Source: CAD feature listing. Evaluate the final solid. Frame: model axes, mm. A direction names the side the tool comes from. Give positions to 0.01 mm unless a question says otherwise; leave off trailing zeros. Write each loop counter-clockwise with the first axis right and the second up, starting at its lowest first coordinate (ties: lowest second). Pieces come first, ordered by that corner, then holes. Notation, with made-up numbers: (14, 53.25) -> (70, 53.25) arc R18 cw to (70, 60.25) -> close; hole circle Ø4 at (38, 78.5). An arc over 180 degrees is marked (long way). Write item = value, one per line.
Autodesk Inventor part; units mm, degrees
ref_plane "Work Plane1" through (18, 0, 0) normal (1, 0, 0) x (0, 1, 0)
ref_plane "Work Plane2" through (0, 0, 5) normal (0, 0, 1) x (1, 0, 0)
ref_plane "XZ Plane" through (0, 0, 0) normal (0, 1, 0) x (-1, 0, 0)
sketch "Sketch1" plane through (0, 0, 0) normal (0, 0, 1) x (1, 0, 0)
  circle A0 centre (0, 0) radius 20
  dimension "d0" = 40
extrude "Extrusion1" add sketch "Sketch1" along normal blind 25
shell "Shell1" thickness 5 removed faces 1 at (-2.364, 6.2334, 25)
fillet "Fillet1" radius 5 1 edges at (-15, 0, 5)
sketch "Sketch2" plane through (0, 0, 0) normal (1, 0, 0) x (0, 1, 0)
  line L0 (-28, 0) -> (28, 0)
  line L1 (0, -5) -> (0, 30)
  circle A0 centre (0, 20) radius 4
  line L2 (20, 25) -> (-20, 25)
  point P0 (0, 0)
  dimension "d5" = 8
  dimension "d6" = 5
extrude "Extrusion2" add sketch "Sketch2" along normal through all both and the other way through all
ref_plane "Work Plane1" through (18, 0, 0) normal (1, 0, 0) x (0, 1, 0)
sketch "Sketch3" plane through (18, 0, 0) normal (1, 0, 0) x (0, 1, 0)
  spline S0 degree 5 poles (4, 20) (4, 20.475) (3.9296, 20.9492) (3.7887, 21.4163) (3.5746, 21.8668) (3.0962, 22.5531) (2.8791, 22.8072) (2.6286, 23.0458) (2.3433, 23.263) (1.6847, 23.649) (1.3023, 23.8174) (0.8849, 23.938) (0.4453, 24) (-0.4453, 24) (-0.8849, 23.938) (-1.3023, 23.8174) (-1.6847, 23.649) (-2.3433, 23.263) (-2.6286, 23.0458) (-2.8791, 22.8072) (-3.0962, 22.5531) (-3.5746, 21.8668) (-3.7887, 21.4163) (-3.9296, 20.9492) (-4, 20.475) (-4, 19.6437) (-3.9603, 19.2875) (-3.881, 18.9346) (-3.7611, 18.5887) (-3.4806, 18.0102) (-3.3396, 17.7723) (-3.1752, 17.5422) (-2.9865, 17.3225) (-2.4836, 16.839) (-2.1457, 16.5837) (-1.7587, 16.3645) (-1.3265, 16.1959) (-0.4314, 15.9995) (0.0204, 15.9613) (0.4754, 15.9901) (0.9122, 16.0827) (1.662, 16.3427) (1.9854, 16.5006) (2.2787, 16.6866) (2.5408, 16.8939) (3.2793, 17.604) (3.6446, 18.1696) (3.8809, 18.7676) (4, 19.3828) (4, 20) knots 0 0 0 0 0 0 0.108769 0.108769 0.108769 0.108769 0.177598 0.177598 0.177598 0.177598 0.250135 0.250135 0.250135 0.250135 0.322672 0.322672 0.322672 0.322672 0.3915 0.3915 0.3915 0.3915 0.50027 0.50027 0.50027 0.50027 0.581861 0.581861 0.581861 0.581861 0.641459 0.641459 0.641459 0.641459 0.721814 0.721814 0.721814 0.721814 0.794745 0.794745 0.794745 0.794745 0.859101 0.859101 0.859101 0.859101 1 1 1 1 1 1
  point P0 (0, 0)
  dimension "d10" = 0
extrude "Extrusion3" cut sketch "Sketch3" along normal through all
mirror "Mirror1" about plane through (0, 0, 0) normal (1, 0, 0) of "Extrusion3"
ref_plane "Work Plane2" through (0, 0, 5) normal (0, 0, 1) x (1, 0, 0)
sketch "Sketch4" plane through (0, 0, 5) normal (0, 0, 1) x (1, 0, 0)
  circle A0 centre (0, 0) radius 15
  circle A1 centre (0, 0) radius 20
  circle A2 centre (0, 0) radius 19
  dimension "d14" = 1
extrude "Extrusion4" cut sketch "Sketch4" along normal blind 1 contours A1
pattern_linear "Rectangular Pattern1" count 3 spacing 2 along (0, 0, 1) of "Extrusion4"
properties part number "Piston" material "Steel, Carbon"
1) Cut plane A-A (z = 13.25). Return the cut outline in (x, y), then the cut area to 3 significant figures.
Computed:
outline = circle Ø40 at (0, 0); hole circle Ø30 at (0, 0)
area = 550 mm²
2) Cut plane D-D (y = 16.5). Return the cut outline in (x, z).
Computed:
outline = (-11.3, 0) -> (11.3, 0) -> (11.3, 5) -> (9.42, 5) -> (9.42, 6) -> (11.3, 6) -> (11.3, 7) -> (9.42, 7) -> (9.42, 8) -> (11.3, 8) -> (11.3, 9) -> (9.42, 9) -> (9.42, 10) -> (11.3, 10) -> (11.3, 25) -> (-11.3, 25) -> (-11.3, 10) -> (-9.42, 10) -> (-9.42, 9) -> (-11.3, 9) -> (-11.3, 8) -> (-9.42, 8) -> (-9.42, 7) -> (-11.3, 7) -> (-11.3, 6) -> (-9.42, 6) -> (-9.42, 5) -> (-11.3, 5) -> close
3) Cut plane C-C (z = 23). State how many separate pieces and enclosed holes the cut face has, then the cut area to 3 significant figures.
Computed:
separate_pieces = 1
enclosed_holes = 2
area = 687 mm²
4) Draft query along X for faces 3 (the cylindrical face through (-4.336, 19.524, 2.465)), 4 (the cylindrical face through (0.21, -0.521, 23.966)), 5 (the flat face through (3, 15, 25)). Return one class per face: pulls with the +X half, pulls with the -X half, needs draft (parallel to the pull), parting line crosses it, or undercut.
Computed:
face_3 = parting line crosses it
face_4 = undercut
face_5 = needs draft
5) Cut plane B-B (y = -17). Return the cut outline in (x, z), then the cut area to 3 significant figures.
Computed:
outline = (-10.54, 0) -> (10.54, 0) -> (10.54, 5) -> (8.49, 5) -> (8.49, 6) -> (10.54, 6) -> (10.54, 7) -> (8.49, 7) -> (8.49, 8) -> (10.54, 8) -> (10.54, 9) -> (8.49, 9) -> (8.49, 10) -> (10.54, 10) -> (10.54, 25) -> (-10.54, 25) -> (-10.54, 10) -> (-8.49, 10) -> (-8.49, 9) -> (-10.54, 9) -> (-10.54, 8) -> (-8.49, 8) -> (-8.49, 7) -> (-10.54, 7) -> (-10.54, 6) -> (-8.49, 6) -> (-8.49, 5) -> (-10.54, 5) -> close
area = 514 mm²
6) Access query for faces 1 (the cylindrical face through (-4.336, 19.524, 6.493)), 2 (the flat face through (18, -7, 7)). Directions: +Z, -Z, +X, -X, +Y, -Y. A direction counts if a zero-diameter tool reaches every point of the face in a straight line with its end or side. Return the directions, or none.
Computed:
face_1 = +Z, -Z
face_2 = none
7) Contact query for flat-ended pins moving along their axis: pin 1 (6 mm diameter, centred on y = -13.5, z = 14.5, fed in from -X); pin 2 (5 mm diameter, centred on y = 7.5, z = 10, fed in from -X); pin 3 (1 mm diameter, centred on x = -3.5, z = 12.5, fed in from +Y). Output: stop coordinate, or through.
Computed:
pin_1 = -17.02
pin_2 = -19.36
pin_3 = 19.77
8) Material intervals for L1, parallel to Z at x = -7.5, y = -18; L2, parallel to Y at x = 0, z = 15.75; L3, parallel to Y at x = -12.5, z = 16.75, sorted ascending.
Computed:
L1 = 0 to 5, 6 to 7, 8 to 9, 10 to 25
L2 = -20 to -15, 15 to 20
L3 = -15.61 to -8.29, -2.33 to 2.33, 8.29 to 15.61
